Here's the drawing with two shaded views (mm, measured from the low corner). I have some questions. A direction names the side the tool comes from. Round coordinates to 2 decimals unless told otherwise and drop trailing zeros. Loops run counter-clockwise (first coordinate to the right, second up) from the corner with the lowest first, then second, coordinate; pieces in that order, holes last. Notation, with made-up numbers: M -19.75,-13 L 38.25,-13 A11 cw 38.25,6 Z; hole C 49.5,-34 d10. An arc over 180 degrees is marked long. Answer as a JSON object with one key per item and string values.
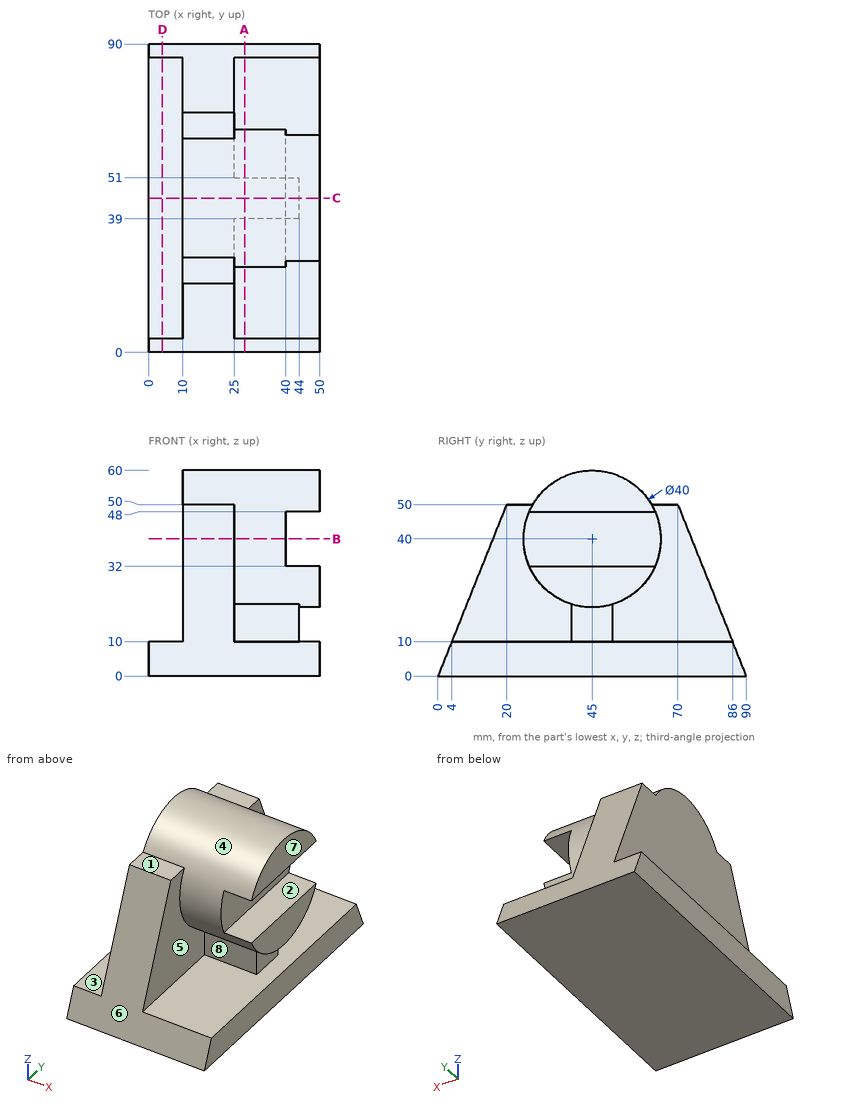
Item 1: I want a section at D-D on x = 4. List the corners of the cut face in (y, z) for me.
Solution:
{"outline": "M 0,0 L 90,0 L 86,10 L 4,10 Z"}
Item 2: I want a section at B-B on z = 40. List the corners of the cut face in (x, y) for me, plus the area to 3 significant figures.
Solution:
{"outline": "M 10,16 L 25,16 L 25,25 L 40,25 L 40,65 L 25,65 L 25,74 L 10,74 Z", "area": "1,470 mm2"}
Item 3: For the marked faces 1, 2, 3, 4 and 5, which set-ups out of +Z, -Z, +X, -X, +Y, -Y let a thin tool reach every point of the face, with its end or its side?
Solution:
{"face 1": "+Z, +X, -X, -Y", "face 2": "+X, +Y, -Y", "face 3": "+Z, -X, +Y, -Y", "face 4": "+X", "face 5": "+X, -Y"}
Item 4: We'd pull the mould along Z, two halves only. Please class the marked faces 6, 7 and 8: +Z half, -Z half, draft (parallel to the pull), parting line (faces both ways), or undercut.
Solution:
{"face 6": "+Z half", "face 7": "draft", "face 8": "undercut"}
Item 5: For P1, Ø17.5, axis at y = 75, z = 26.5, coming from the +X side; P2, Ø15, axis at y = 36, z = 39.5, coming from the -X side; P3, Ø13, axis at y = 54.5, z = 40, coming from the +X side, each with a flat end and sliding along its axis, tell me the tip position at first contact or that it passes through.
Solution:
{"P1": "stops at x = 25", "P2": "stops at x = 10", "P3": "stops at x = 40"}
Item 6: I want a section at A-A on x = 28. List the corners of the cut face in (y, z) for me, plus the area to 3 significant figures.
Solution:
{"outline": "M 0,0 L 90,0 L 86,10 L 51,10 L 51,20.92 A20 ccw long 39,20.92 L 39,10 L 4,10 Z", "area": "2,240 mm2"}
Item 7: If I drill on L1, parallel to Z at x = 27, y = 77.5; L2, parallel to Z at x = 41, y = 62; L3, parallel to X at y = 80, z = 14, over which ranges is the centre line in solid material (lowest first)? Write a range as from..to.
Solution:
{"L1": "z = 0..10", "L2": "z = 0..10, 29.46..32, 48..50.54", "L3": "x = 10..25"}
Item 8: I want a section at C-C on y = 45. List the corners of the cut face in (x, z) for me, plus the area to 3 significant figures.
Solution:
{"outline": "M 0,0 L 50,0 L 50,10 L 44,10 L 44,20 L 50,20 L 50,32 L 40,32 L 40,48 L 50,48 L 50,60 L 10,60 L 10,10 L 0,10 Z", "area": "2,280 mm2"}
